```python
from build123d import *

# Parameters (mm, degrees)
BOSS_EXTRUDE1_DEPTH = 15
CUT_EXTRUDE1_DEPTH  = 136.508273532
SKETCH3_R           = 2
CUT_EXTRUDE2_DEPTH  = 136.508273532
SKETCH4_R           = 1.6
CUT_EXTRUDE3_DEPTH  = 135.898080771
FILLET1_R           = 5
FILLET2_R           = 7
SKETCH6_R           = 3.5
CUT_EXTRUDE4_DEPTH  = 3
SKETCH7_R           = 1
CUT_EXTRUDE5_DEPTH  = 5


with BuildPart() as part:
    # Sketch1 → Boss-Extrude1 (new body)
    with BuildSketch(Plane(origin=(0, 0, 0), x_dir=(1, 0, 0), z_dir=(0, 1, 0))):
        with BuildLine():
            Line((-30.483870968, -13.842203604), (-30.483870968, -17.842203604))
            Line((-30.483870968, -17.842203604), (-15.483870968, -17.842203604))
            Line((-15.483870968, -17.842203604), (-11.604336021, -17.842203604))
            ThreePointArc((-11.604336021, -17.842203604), (-10.652040513, -18.537026173), (-11.023097827, -19.655937075))
            Line((-11.023097827, -19.655937075), (-14.180005266, -21.91087096))
            ThreePointArc((-14.180005266, -21.91087096), (-15.56030908, -22.603681147), (-17.086196235, -22.842203604))
            Line((-17.086196235, -22.842203604), (-30.483870968, -22.842203604))
            Line((-30.483870968, -22.842203604), (-30.483870968, -26.842203604))
            Line((-30.483870968, -26.842203604), (-14.306659767, -26.842203604))
            ThreePointArc((-14.306659767, -26.842203604), (-12.714208629, -26.581834325), (-11.287607633, -25.827843353))
            Line((-11.287607633, -25.827843353), (-2.084385084, -18.856563855))
            ThreePointArc((-2.084385084, -18.856563855), (-0.657784088, -18.102572883), (0.93466705, -17.842203604))
            Line((0.93466705, -17.842203604), (90.131209208, -17.842203604))
            ThreePointArc((90.131209208, -17.842203604), (91.465877117, -18.023628963), (92.703687985, -18.554738975))
            Line((92.703687985, -18.554738975), (100.32857008, -23.129668233))
            ThreePointArc((100.32857008, -23.129668233), (101.566380948, -23.660778245), (102.901048857, -23.842203604))
            Line((102.901048857, -23.842203604), (131.516129032, -23.842203604))
            Line((131.516129032, -23.842203604), (131.516129032, -13.842203604))
            Line((131.516129032, -13.842203604), (117.516129032, -13.842203604))
            ThreePointArc((117.516129032, -13.842203604), (116.809022251, -13.549310385), (116.516129032, -12.842203604))
            Line((116.516129032, -12.842203604), (116.516129032, -4.842203604))
            ThreePointArc((116.516129032, -4.842203604), (116.809022251, -4.135096823), (117.516129032, -3.842203604))
            Line((117.516129032, -3.842203604), (131.516129032, -3.842203604))
            Line((131.516129032, -3.842203604), (131.516129032, -0.842203604))
            Line((131.516129032, -0.842203604), (131.516129032, 2.157796396))
            Line((131.516129032, 2.157796396), (112.422801941, 2.157796396))
            ThreePointArc((112.422801941, 2.157796396), (111.530677914, 2.077564147), (110.667184733, 1.839442284))
            Line((110.667184733, 1.839442284), (104.365073331, -0.523849492))
            ThreePointArc((104.365073331, -0.523849492), (103.501580151, -0.761971355), (102.609456123, -0.842203604))
            Line((102.609456123, -0.842203604), (-30.483870968, -0.842203604))
            Line((-30.483870968, -0.842203604), (-30.483870968, -4.842203604))
            Line((-30.483870968, -4.842203604), (-10.483870968, -4.842203604))
            ThreePointArc((-10.483870968, -4.842203604), (-9.069657405, -5.427990042), (-8.483870968, -6.842203604))
            Line((-8.483870968, -6.842203604), (-8.483870968, -11.842203604))
            ThreePointArc((-8.483870968, -11.842203604), (-9.069657405, -13.256417166), (-10.483870968, -13.842203604))
            Line((-10.483870968, -13.842203604), (-30.483870968, -13.842203604))
        make_face()
        with BuildLine():
            Line((-3.483870968, -4.842203604), (27.516129032, -4.842203604))
            ThreePointArc((27.516129032, -4.842203604), (28.223235813, -5.135096823), (28.516129032, -5.842203604))
            Line((28.516129032, -5.842203604), (28.516129032, -12.336203873))
            ThreePointArc((28.516129032, -12.336203873), (28.223235813, -13.043310655), (27.516129032, -13.336203873))
            Line((27.516129032, -13.336203873), (-3.483870968, -13.336203873))
            ThreePointArc((-3.483870968, -13.336203873), (-4.190977749, -13.043310655), (-4.483870968, -12.336203873))
            Line((-4.483870968, -12.336203873), (-4.483870968, -5.842203604))
            ThreePointArc((-4.483870968, -5.842203604), (-4.190977749, -5.135096823), (-3.483870968, -4.842203604))
        make_face(mode=Mode.SUBTRACT)
        with BuildLine():
            Line((32.516129032, -4.842203604), (55.516129032, -4.842203604))
            ThreePointArc((55.516129032, -4.842203604), (56.223235813, -5.135096823), (56.516129032, -5.842203604))
            Line((56.516129032, -5.842203604), (56.516129032, -12.336203873))
            ThreePointArc((56.516129032, -12.336203873), (56.223235813, -13.043310655), (55.516129032, -13.336203873))
            Line((55.516129032, -13.336203873), (32.516129032, -13.336203873))
            ThreePointArc((32.516129032, -13.336203873), (31.809022251, -13.043310655), (31.516129032, -12.336203873))
            Line((31.516129032, -12.336203873), (31.516129032, -5.842203604))
            ThreePointArc((31.516129032, -5.842203604), (31.809022251, -5.135096823), (32.516129032, -4.842203604))
        make_face(mode=Mode.SUBTRACT)
        with BuildLine():
            Line((60.516129032, -4.842203604), (83.516129032, -4.842203604))
            ThreePointArc((83.516129032, -4.842203604), (84.223235813, -5.135096823), (84.516129032, -5.842203604))
            Line((84.516129032, -5.842203604), (84.516129032, -12.336203873))
            ThreePointArc((84.516129032, -12.336203873), (84.223235813, -13.043310655), (83.516129032, -13.336203873))
            Line((83.516129032, -13.336203873), (60.516129032, -13.336203873))
            ThreePointArc((60.516129032, -13.336203873), (59.809022251, -13.043310655), (59.516129032, -12.336203873))
            Line((59.516129032, -12.336203873), (59.516129032, -5.842203604))
            ThreePointArc((59.516129032, -5.842203604), (59.809022251, -5.135096823), (60.516129032, -4.842203604))
        make_face(mode=Mode.SUBTRACT)
        with BuildLine():
            Line((88.516129032, -4.842203604), (111.516129032, -4.842203604))
            ThreePointArc((111.516129032, -4.842203604), (112.223235813, -5.135096823), (112.516129032, -5.842203604))
            Line((112.516129032, -5.842203604), (112.516129032, -12.336203873))
            ThreePointArc((112.516129032, -12.336203873), (112.223235813, -13.043310655), (111.516129032, -13.336203873))
            Line((111.516129032, -13.336203873), (88.516129032, -13.336203873))
            ThreePointArc((88.516129032, -13.336203873), (87.809022251, -13.043310655), (87.516129032, -12.336203873))
            Line((87.516129032, -12.336203873), (87.516129032, -5.842203604))
            ThreePointArc((87.516129032, -5.842203604), (87.809022251, -5.135096823), (88.516129032, -4.842203604))
        make_face(mode=Mode.SUBTRACT)
    extrude(amount=BOSS_EXTRUDE1_DEPTH)

    # Sketch2 → Cut-Extrude1 (cut, through all)
    with BuildSketch(Plane.XY.offset(26.842203604)):
        Polygon((-14.306659767, 2.215189944), (-30.483870968, 2.5), (-30.483870968, 0), (-14.306659767, 0), align=None)
        Polygon((111.516129032, 0), (-14.306659767, 2.215189944), (-14.306659767, 0), align=None)
        Polygon((-30.483870968, 15), (-30.483870968, 12.5), (-14.306659767, 12.784810056), (-14.306659767, 15), align=None)
        Polygon((-14.306659767, 15), (-14.306659767, 12.784810056), (111.516129032, 15), align=None)
    extrude(amount=-CUT_EXTRUDE1_DEPTH, mode=Mode.SUBTRACT)

    # Sketch3 → Cut-Extrude2 (cut, through all)
    with BuildSketch(Plane.XY.offset(26.842203604)):
        with Locations((-25.483870968, 7.5)):
            Circle(SKETCH3_R)
    extrude(amount=-CUT_EXTRUDE2_DEPTH, mode=Mode.SUBTRACT)

    # Sketch4 → Cut-Extrude3 (cut, through all)
    with BuildSketch(Plane.XY.offset(23.842203604)):
        with Locations((124.516129032, 7.5)):
            Circle(SKETCH4_R)
    extrude(amount=-CUT_EXTRUDE3_DEPTH, mode=Mode.SUBTRACT)

    # Fillet1
    fillet1_edges = [part.edges().sort_by_distance(p)[0] for p in [
        (-30.483870968, 2.5, 2.842203604),
        (-30.483870968, 2.5, 15.842203604),
        (-30.483870968, 2.5, 24.842203604),
        (-30.483870968, 12.5, 2.842203604),
        (-30.483870968, 12.5, 15.842203604),
        (-30.483870968, 12.5, 24.842203604),
    ]]
    fillet(fillet1_edges, radius=FILLET1_R)

    # Fillet2
    fillet2_edges = [part.edges().sort_by_distance(p)[0] for p in [
        (131.516129032, 0, 0.842203604),
        (131.516129032, 0, 18.842203604),
        (131.516129032, 15, 18.842203604),
        (131.516129032, 15, 0.842203604),
    ]]
    fillet(fillet2_edges, radius=FILLET2_R)

    # Sketch6 → Cut-Extrude4 (cut)
    with BuildSketch(Plane.XY.offset(23.842203604)):
        with Locations((124.516129032, 7.5)):
            Circle(SKETCH6_R)
    extrude(amount=-CUT_EXTRUDE4_DEPTH, mode=Mode.SUBTRACT)

    # Sketch7 → Cut-Extrude5 (cut)
    with BuildSketch(Plane.XY.offset(23.842203604)):
        with Locations((111.516129032, 7.5)):
            Circle(SKETCH7_R)
    extrude(amount=-CUT_EXTRUDE5_DEPTH, mode=Mode.SUBTRACT)


solid = part.part
```
Geometry check sheet. Reference: the model listing, model coordinates, mm. A direction names the side the tool comes from. Coordinates: 2 decimals unless noted, no trailing zeros. Order: outer loops, then holes, each group sorted by start corner. A loop starts at its lowest first (then second) coordinate and runs counter-clockwise, first axis right, second up. Notation, with made-up numbers: M -16.5,61 L 21.5,61 A5 cw 21.5,65 Z; hole C 71.25,1.25 d1. An arc over 180 degrees is marked long. Answer as a JSON object with one key per item and string values.
Q1. Cross-section at C-C on x = 98. Record the cut outline in (y, z).
Results are:
{"outline": "M 0.24,0.84 L 14.76,0.84 L 14.76,4.84 L 0.24,4.84 Z; M 0.24,13.34 L 14.76,13.34 L 14.76,21.73 L 0.24,21.73 Z"}
Q2. Depth check by flat-ended pin: pin 1 Ø1.9 at (y, z) = (6, 8) entering from -X; pin 2 Ø8 at (x, z) = (63.5, 16) entering from +Y; pin 3 Ø12 at (x, z) = (-10, 7) entering from -Y; pin 4 Ø2.5 at (x, y) = (124.52, 7.5) entering from +Z. Enter the tip coordinate at first touch or a pass-through.
Results are:
{"pin 1": "stops at x = -8.48", "pin 2": "stops at y = 14.23", "pin 3": "stops at y = 2.04", "pin 4": "passes through"}
Q3. Release check for a two-part mould opening along Z. For faces 1 (the flat face through (44, 7, 13.336)), 2 (the flat face through (28.516, 7, 9)), 3 (the cylindrical face through (129.411, 13.004, 0.8)), 4 (the cylindrical face through (101.548, 7.397, 23.656)) record: released by +Z, released by -Z, zero draft, split by the parting line, or undercut.
Results are:
{"face 1": "undercut", "face 2": "undercut", "face 3": "zero draft", "face 4": "released by +Z"}
Q4. Tool access check on faces 5 (the cylindrical face through (91.45, 7.4, 18.02)), 6 (the flat face through (117, 7, 23.842)), 7 (the flat face through (84.516, 7, 9)), 8 (the flat face through (-20, 7, 13.842)). Record the directions out of +Z, -Z, +X, -X, +Y, -Y that give a thin tool (end or side, any length) a straight path to the whole face; none if there is none.
Results are:
{"face 5": "+Z, +Y, -Y", "face 6": "+Z, +X, +Y, -Y", "face 7": "+Y, -Y", "face 8": "-X, +Y, -Y"}
Q5. Cross-section at A-A on z = 10.5. Record the cut outline in (x, y).
Results are:
{"outline": "M -8.48,2.11 L -4.48,2.04 L -4.48,12.96 L -8.48,12.89 Z; M 28.52,1.46 L 31.52,1.41 L 31.52,13.59 L 28.52,13.54 Z; M 56.52,0.97 L 59.52,0.92 L 59.52,14.08 L 56.52,14.03 Z; M 84.52,0.48 L 87.52,0.42 L 87.52,14.58 L 84.52,14.52 Z; M 112.52,0 L 116.52,0 L 116.52,15 L 112.52,15 Z"}
Q6. Cross-section at B-B on x = 68. Record the cut outline in (y, z).
Results are:
{"outline": "M 0.77,0.84 L 14.23,0.84 L 14.23,4.84 L 0.77,4.84 Z; M 0.77,13.34 L 14.23,13.34 L 14.23,17.84 L 0.77,17.84 Z"}
Q7. Scan lines: line 1 (Z direction, x = -17, y = 9.25); line 2 (X direction, y = 8.5, z = 10.25); line 3 (Z direction, x = 40, y = 9). Record each from-to range of solid material in increasing order.
Results are:
{"line 1": "z = 0.84 to 4.84, 13.84 to 17.84, 22.84 to 26.84", "line 2": "x = -8.48 to -4.48, 28.52 to 31.52, 56.52 to 59.52, 84.52 to 87.52, 112.52 to 116.52", "line 3": "z = 0.84 to 4.84, 13.34 to 17.84"}
